```python
from build123d import *

# Parameters (mm, degrees)
ESQUISSE1_W             = 8
ESQUISSE1_H             = 15
CHANFREIN1_SIZE         = 1
ESQUISSE3_R             = 2
ESQUISSE3_R_2           = 2.5
ENL_V_MAT_EXTRU_2_DEPTH = 51.139804547


with BuildPart() as part:
    # Esquisse1 → Base-Révolution (revolve)
    with BuildSketch(Plane.XY, mode=Mode.PRIVATE) as base_r_volution_sk:
        with Locations((4, 27.5)):
            Rectangle(ESQUISSE1_W, ESQUISSE1_H)
    revolve(base_r_volution_sk.sketch.rotate(Axis((0, 0, 0), (1, 0, 0)), 90), axis=Axis((0, 0, 0), (1, 0, 0)))

    # Chanfrein1
    chanfrein1_edges = [part.edges().sort_by_distance(p)[0] for p in [
        (0, 0, -35),
        (8, 0, -35),
    ]]
    chamfer(chanfrein1_edges, length=CHANFREIN1_SIZE)

    # Esquisse3 → Enlèv. mat.-Extru.2 (cut, through all)
    with BuildSketch(Plane.ZY):
        with Locations((0, 30)):
            Circle(ESQUISSE3_R)
        with Locations((21.213203436, 21.213203436)):
            Circle(ESQUISSE3_R_2)
        with Locations((30, 0)):
            Circle(ESQUISSE3_R)
        with Locations((21.213203436, -21.213203436)):
            Circle(ESQUISSE3_R_2)
        with Locations((0, -30)):
            Circle(ESQUISSE3_R)
        with Locations((-21.213203436, -21.213203436)):
            Circle(ESQUISSE3_R_2)
        with Locations((-30, 0)):
            Circle(ESQUISSE3_R)
        with Locations((-21.213203436, 21.213203436)):
            Circle(ESQUISSE3_R_2)
    extrude(amount=-ENL_V_MAT_EXTRU_2_DEPTH, mode=Mode.SUBTRACT)


solid = part.part
```
Here's how the part is built. I have some questions about the finished solid (model axes, mm). Coordinates: 2 decimals unless noted, no trailing zeros. Order: outer loops, then holes, each group sorted by start corner. A loop starts at its lowest first (then second) coordinate and runs counter-clockwise, first axis right, second up. Notation, with made-up numbers: M 45,76 L 49,76 A22 ccw 49,101 Z; hole C 71,83.25 d8. An arc over 180 degrees is marked long. Answer as a JSON object with one key per item and string values. Group by question number.
(1) For pin 1 (1 mm diameter, centred on x = 6.5, y = 22, fed in from -Z); pin 2 (3 mm diameter, centred on y = -21.21, z = -21.21, fed in from -X); pin 3 (6 mm diameter, centred on y = 21.21, z = -21.21, fed in from -X); pin 4 (3 mm diameter, centred on x = 6, y = -23.5, fed in from -Z), each with a flat end and sliding along its axis, tell me the tip position at first contact or that it passes through.
(2) Suppose I cut it at A-A, the plane y = 0. Please give me the cut outline in (x, z), then the cut area to 3 significant figures.
(3) Suppose I cut it at B-B, the plane x = 5.5. State how many separate pieces and enclosed holes the cut face has, then the cut area to 3 significant figures.
(4) If we mould it in two halves opening along Z, with no side actions, what happens to faces 1 (the face through (3.944, 0.601, -28.092)), 2 (the face through (4.042, 34.168, -7.587)), 3 (the face through (8, 15, -15)), 4 (the face through (3.944, 0.601, 31.908))? For each: released by +Z, released by -Z, zero draft, split by the parting line, or undercut.
(5) I need wall thicknesses on probe 1 along Y at (x, z) = (1.5, 0); probe 2 along Z at (x, y) = (6.5, -1.5); probe 3 along Y at (x, z) = (5, -23.5). Which ranges of each line are inside material? Lowest first, please.
Values found:
{
 "1": {"pin 1": "stops at z = -27.62", "pin 2": "passes through", "pin 3": "stops at x = 0", "pin 4": "stops at z = -27.22"},
 "2": {"outline": "M 0,-34 L 1,-35 L 7,-35 L 8,-34 L 8,-32 L 0,-32 Z; M 0,-28 L 8,-28 L 8,-20 L 0,-20 Z; M 0,20 L 8,20 L 8,28 L 0,28 Z; M 0,32 L 8,32 L 8,34 L 7,35 L 1,35 L 0,34 Z", "area": "174 mm^2"},
 "3": {"separate pieces": "1", "enclosed holes": "9", "area": "2,460 mm^2"},
 "4": {"face 1": "undercut", "face 2": "split by the parting line", "face 3": "zero draft", "face 4": "undercut"},
 "5": {"probe 1": "y = -35 to -32, -28 to -20, 20 to 28, 32 to 35", "probe 2": "z = -34.97 to -31.32, -28.68 to -19.94, 19.94 to 28.68, 31.32 to 34.97", "probe 3": "y = -25.94 to -22.22, -20.2 to 20.2, 22.22 to 25.94"}
}
